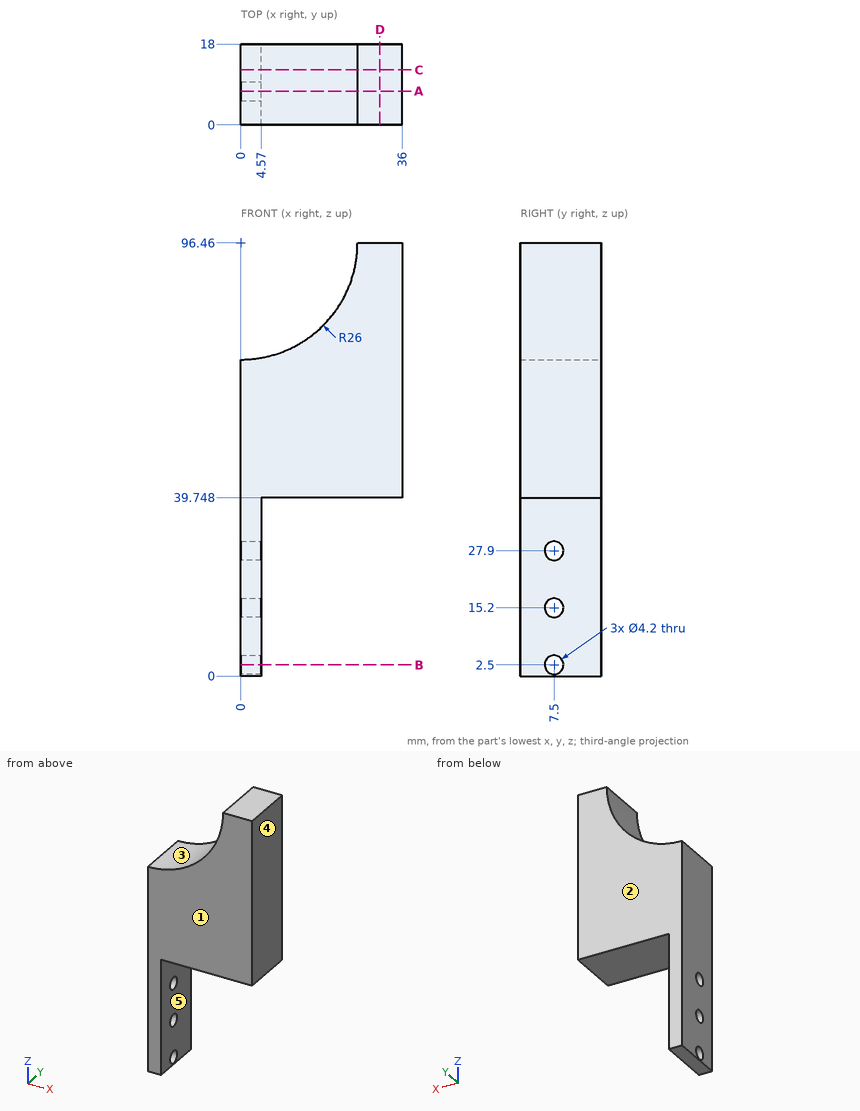
Could you check a few things on this drawing? It's one solid part, dimensions in mm from its lowest x, y, z. A direction names the side the tool comes from. Coordinates: 2 decimals unless noted, no trailing zeros. Write each loop counter-clockwise with the first axis right and the second up, starting at its lowest first coordinate (ties: lowest second). Pieces come first, ordered by that corner, then holes.
1) Which directions (+Z, -Z, +X, -X, +Y, -Y) give clear straight access to the entire face, cutting with the end or side of a thin tool? Please do the marked faces 4 and 5.
Filled in:
face 4: +Z, -Z, +X, +Y, -Y
face 5: -Z, +X, +Y, -Y
2) If I drill on line 1 (Y direction, x = 1.2, z = 2.5); line 2 (X direction, y = 7.25, z = 25); line 3 (Z direction, x = 34, y = 15.5), over which ranges is the centre line in solid material (lowest first)?
Filled in:
line 1: y = 0 to 5.4, 9.6 to 18
line 2: x = 0 to 4.57
line 3: z = 39.75 to 96.46
3) If we section it at A-A (y = 7.5): List the corners of the cut face in (x, z) for me, plus the area to 3 significant figures.
Filled in:
outline: (0, 0) - (4.57, 0) - (4.57, 0.4) - (0, 0.4) - close; (0, 4.6) - (4.57, 4.6) - (4.57, 13.1) - (0, 13.1) - close; (0, 17.3) - (4.57, 17.3) - (4.57, 25.8) - (0, 25.8) - close; (0, 30) - (4.57, 30) - (4.57, 39.75) - (36, 39.75) - (36, 96.46) - (26, 96.46) arc R26 cw to (0, 70.46) - close
area: 1,630 mm2
4) If we section it at C-C (y = 12.25): List the corners of the cut face in (x, z) for me, plus the area to 3 significant figures.
Filled in:
outline: (0, 0) - (4.57, 0) - (4.57, 39.75) - (36, 39.75) - (36, 96.46) - (26, 96.46) arc R26 cw to (0, 70.46) - close
area: 1,690 mm2
5) If we section it at B-B (z = 2.5): List the corners of the cut face in (x, y) for me, plus the area to 3 significant figures.
Filled in:
outline: (0, 0) - (4.57, 0) - (4.57, 5.4) - (0, 5.4) - close; (0, 9.6) - (4.57, 9.6) - (4.57, 18) - (0, 18) - close
area: 63.1 mm2
6) If we section it at D-D (x = 31): List the corners of the cut face in (y, z) for me, plus the area to 3 significant figures.
Filled in:
outline: (0, 39.75) - (18, 39.75) - (18, 96.46) - (0, 96.46) - close
area: 1,020 mm2
7) Thinking about a two-plate mould opening in Y: for the marked faces 1, 2 and 3, which applies, +Y half, -Y half, draft (parallel to the pull), parting line (faces both ways), or undercut?
Filled in:
face 1: -Y half
face 2: +Y half
face 3: draft
8) I'm going to push flat-ended pins straight in: pin 1 (6 mm diameter, centred on y = 8.5, z = 11, fed in from +X); pin 2 (3.5 mm diameter, centred on y = 7.5, z = 2.5, fed in from -X); pin 3 (1 mm diameter, centred on y = 14.5, z = 84, fed in from -X); pin 4 (1 mm diameter, centred on y = 8.5, z = 19.5, fed in from -X). Where does each tip first touch, or does it pass through?
Filled in:
pin 1: stops at x = 4.57
pin 2: passes through
pin 3: stops at x = 22.54
pin 4: stops at x = 0
